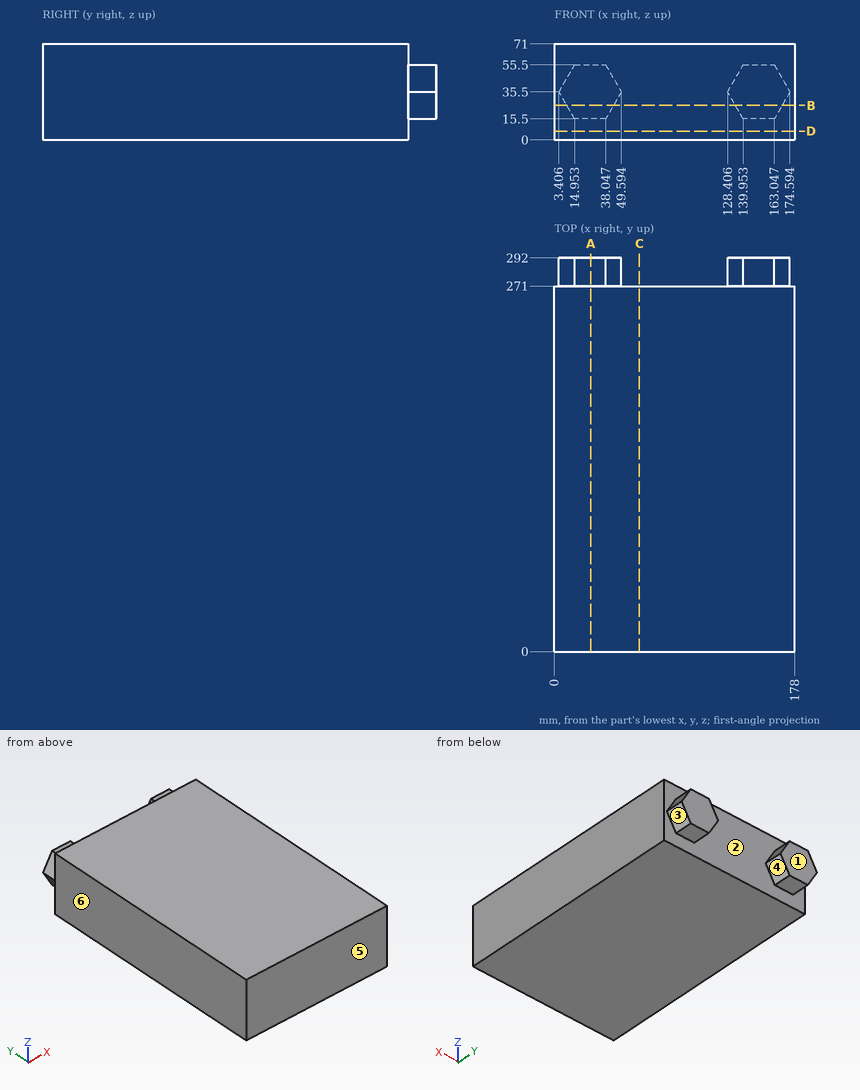
Job drawing, mm, ordinate dimensions from the low corner. One solid piece. A direction names the side the tool comes from. Round coordinates to 2 decimals unless told otherwise and drop trailing zeros. Loops run counter-clockwise (first coordinate to the right, second up) from the corner with the lowest first, then second, coordinate; pieces in that order, holes last. Notation, with made-up numbers: (7.25, 53) -> (66.25, 53) arc R32 ccw to (66.25, 92) -> close; hole circle Ø11 at (61, 63.5). An arc over 180 degrees is marked (long way). Use a Markdown table: item, result.
1) Cut at C-C, the plane x = 63. List the corners of the cut face in (y, z).
The answers:
| item | result |
|---|---|
| outline | (0, 0) -> (271, 0) -> (271, 71) -> (0, 71) -> close |
2) Tool access for the marked faces 1, 2 and 3: list every direction of +Z, -Z, +X, -X, +Y, -Y with a clear straight run to the whole face (end or side of a thin tool).
The answers:
| item | result |
|---|---|
| face 1 | +Z, -Z, +X, -X, +Y |
| face 2 | +Y |
| face 3 | -Z, +X, +Y |
3) Drop flat-ended pins along their axis: pin 1 Ø10.5 at (x, y) = (24.5, 284.5) entering from -Z; pin 2 Ø6.5 at (x, y) = (28.5, 286) entering from +Z; pin 3 Ø10 at (x, z) = (89, 47.5) entering from +Y. Give the stop position or say it passes through.
The answers:
| item | result |
|---|---|
| pin 1 | stops at z = 15.5 |
| pin 2 | stops at z = 55.5 |
| pin 3 | stops at y = 271 |
4) Cut at B-B, the plane z = 25.5. List the corners of the cut face in (x, y).
The answers:
| item | result |
|---|---|
| outline | (0, 0) -> (178, 0) -> (178, 271) -> (168.82, 271) -> (168.82, 292) -> (134.18, 292) -> (134.18, 271) -> (43.82, 271) -> (43.82, 292) -> (9.18, 292) -> (9.18, 271) -> (0, 271) -> close |
5) Cut at D-D, the plane z = 6.5. List the corners of the cut face in (x, y).
The answers:
| item | result |
|---|---|
| outline | (0, 0) -> (178, 0) -> (178, 271) -> (0, 271) -> close |
6) Probe line 1 (Y direction, x = 80, z = 26). List the from-to ranges inside material, lowest first. Write a range as [from, to].
The answers:
| item | result |
|---|---|
| line 1 | y = [0, 271] |
7) Pull direction X, two halves, no side cores. Call the marked faces 4, 5 and 6: pulls with the +X half, pulls with the -X half, needs draft (parallel to the pull), parting line crosses it, or undercut.
The answers:
| item | result |
|---|---|
| face 4 | undercut |
| face 5 | needs draft |
| face 6 | pulls with the -X half |
8) Cut at A-A, the plane x = 27. List the corners of the cut face in (y, z), and give its area (3 significant figures).
The answers:
| item | result |
|---|---|
| outline | (0, 0) -> (271, 0) -> (271, 15.5) -> (292, 15.5) -> (292, 55.5) -> (271, 55.5) -> (271, 71) -> (0, 71) -> close |
| area | 20,100 mm2 |
